Part model, mm, in its own coordinate system. Give positions to 0.01 mm unless a question says otherwise; leave off trailing zeros. Write each loop counter-clockwise with the first axis right and the second up, starting at its lowest first coordinate (ties: lowest second). Pieces come first, ordered by that corner, then holes. Notation, with made-up numbers: (50.5, 70) - (103.5, 70) arc R26 cw to (103.5, 93) - close; hole circle Ø9 at (-3.5, 52.25). An arc over 180 degrees is marked (long way). Answer as a JSON object with one key per item and string values. Group by question number.
Autodesk Inventor part; units mm, degrees
ref_plane "YZ Plane" through (0, 0, 0) normal (1, 0, 0) x (0, 1, 0)
ref_plane "XZ Plane" through (0, 0, 0) normal (0, 1, 0) x (-1, 0, 0)
ref_plane "XY Plane" through (0, 0, 0) normal (0, 0, 1) x (1, 0, 0)
sketch "Sketch1" plane through (0, 0, 0) normal (0, 1, 0) x (-1, 0, 0)
  line L0 (717.55, -717.55) -> (-717.55, -717.55)
  line L1 (-717.55, -717.55) -> (-717.55, 717.55)
  line L2 (-717.55, 717.55) -> (717.55, 717.55)
  line L3 (717.55, 717.55) -> (717.55, -717.55)
  line L4 (717.55, -717.55) -> (-717.55, 717.55) construction
  line L5 (-717.55, -717.55) -> (717.55, 717.55) construction
  line L6 (-708.025, -708.025) -> (708.025, -708.025)
  line L7 (708.025, -708.025) -> (708.025, 708.025)
  line L8 (708.025, 708.025) -> (-708.025, 708.025)
  line L9 (-708.025, 708.025) -> (-708.025, -708.025)
  line L10 (701.675, -701.675) -> (-701.675, -701.675)
  line L11 (-701.675, -701.675) -> (-701.675, 701.675)
  line L12 (-701.675, 701.675) -> (701.675, 701.675)
  line L13 (701.675, 701.675) -> (701.675, -701.675)
  point P0 (0, 0)
  dimension "d0" = 1435.1
  dimension "d1" = 1435.1
  dimension "d2" = 9.525
  dimension "d3" = 6.35
extrude "Extrusion1" add sketch "Sketch1" along normal blind 215.9 contours L0 L1 L2 L3 | L9 L8 L7 L6 | L10 L11 L12 L13
sketch "Sketch2" plane through (-717.55, 0, 717.55) normal (0, 0, 1) x (1, 0, 0)
  line L0 (0, 0) -> (1435.1, 0)
  line L1 (1435.1, 0) -> (1435.1, 215.9)
  line L2 (0, 215.9) -> (1435.1, 215.9)
  line L3 (0, 0) -> (0, 215.9)
  line L4 (0, 215.9) -> (1435.1, 215.9)
  line L5 (717.55, 215.9) -> (0, 209.55)
  line L6 (0, 215.9) -> (0, 209.55)
  line L7 (0, 0) -> (0, 215.9)
  line L8 (0, 215.9) -> (717.55, 215.9)
  line L9 (717.55, 215.9) -> (1435.1, 215.9)
  line L10 (1435.1, 0) -> (1435.1, 215.9)
  line L11 (1435.1, 215.9) -> (1435.1, 209.55)
  line L12 (1435.1, 209.55) -> (717.55, 215.9)
  point P0 (717.55, 0)
  dimension "d6" = 6.35
  dimension "d7" = 6.35
sketch "Sketch3" plane through (717.55, 0, 717.55) normal (1, 0, 0) x (0, 0, -1)
  line L0 (0, 0) -> (1435.1, 0)
  line L1 (1435.1, 0) -> (1435.1, 215.9)
  line L2 (0, 215.9) -> (1435.1, 215.9)
  line L3 (0, 0) -> (0, 215.9)
  line L4 (0, 215.9) -> (1435.1, 215.9)
  line L5 (717.55, 215.9) -> (0, 209.55)
  line L6 (0, 0) -> (0, 215.9)
  line L7 (0, 215.9) -> (0, 209.55)
  line L8 (0, 215.9) -> (717.55, 215.9)
  line L9 (717.55, 215.9) -> (1435.1, 215.9)
  line L10 (1435.1, 0) -> (1435.1, 215.9)
  line L11 (1435.1, 215.9) -> (1435.1, 209.55)
  line L12 (1435.1, 209.55) -> (717.55, 215.9)
  point P0 (717.55, 0)
  point P1 (0, 209.55)
  dimension "d8" = 6.35
  dimension "d9" = 6.35
extrude "Extrusion2" cut sketch "Sketch2" against normal through all contours L3 L2 L5 | L12 L2 L1
extrude "Extrusion3" cut sketch "Sketch3" against normal through all contours L3 L2 L5 | L12 L2 L1
extrude "Extrusion4" cut sketch "Sketch1" along normal blind 19.05 contours L9 L8 L7 L6
extrude "Extrusion5" cut sketch "Sketch1" along normal blind 12.7
properties part number "D - Cap - 2" material "Granite, Cut, Polished"
1) Band-saw the part on A-A (x = 439). List the corners of the cut face in (y, z) (3 decimals).
2) Probe line 1 (Y direction, x = 30.5, z = 40); line 2 (Y direction, x = -455, z = -620). List the from-to ranges inside material, lowest first.
3) Band-saw the part on B-B (z = -508.5). List the corners of the cut face in (x, y) (3 decimals).
4) Drop flat-ended pins along their axis: P1, Ø1, axis at x = -385, z = -364, coming from the +Y side; P2, Ø3, axis at x = -108.5, z = -377, coming from the +Y side. Give the stop position or say it passes through.
Verdict:
{
 "1": {"outline": "(12.7, -717.55) - (209.55, -717.55) - (212.015, -439) - (212.015, 439) - (209.55, 717.55) - (12.7, 717.55) - (12.7, 708.025) - (19.05, 708.025) - (19.05, 701.675) - (12.7, 701.675) - (12.7, -701.675) - (19.05, -701.675) - (19.05, -708.025) - (12.7, -708.025) - close"},
 "2": {"line 1": "12.7 to 215.55", "line 2": "12.7 to 210.41"},
 "3": {"outline": "(-717.55, 12.7) - (-708.025, 12.7) - (-708.025, 19.05) - (-701.675, 19.05) - (-701.675, 12.7) - (701.675, 12.7) - (701.675, 19.05) - (708.025, 19.05) - (708.025, 12.7) - (717.55, 12.7) - (717.55, 209.55) - (508.5, 211.4) - (-508.5, 211.4) - (-717.55, 209.55) - close"},
 "4": {"P1": "y = 212.5", "P2": "y = 212.58"}
}
